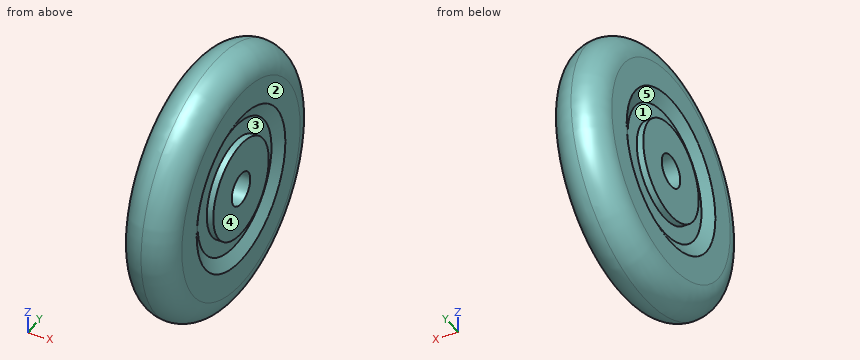
```python
from build123d import *


with BuildPart() as f1:
    # F0 (on Front) → F1 (revolve)
    with BuildSketch(Plane.XZ):
        with BuildLine():
            Line((-12.7, 7.9375), (0, 7.9375))
            Line((0, 7.9375), (12.7, 7.9375))
            Line((12.7, 7.9375), (12.7, 23.8125))
            Line((12.7, 23.8125), (9.525, 23.8125))
            Line((9.525, 23.8125), (9.525, 31.75))
            Line((9.525, 31.75), (12.7, 38.1))
            Line((12.7, 38.1), (12.7, 50.8))
            ThreePointArc((12.7, 50.8), (8.980256, 59.780256), (0, 63.5))
            ThreePointArc((0, 63.5), (-8.980256, 59.780256), (-12.7, 50.8))
            Line((-12.7, 50.8), (-12.7, 38.1))
            Line((-12.7, 38.1), (-9.525, 31.75))
            Line((-9.525, 31.75), (-9.525, 23.8125))
            Line((-9.525, 23.8125), (-12.7, 23.8125))
            Line((-12.7, 23.8125), (-12.7, 7.9375))
        make_face()
    revolve(axis=Axis((-3.268924, 0, 0), (1, 0, 0)))


solid = f1.part
```
Geometry check sheet. Reference: the model listing, model coordinates, mm. Face numbers are marked on the shaded views. A direction names the side the tool comes from. Give positions to 0.01 mm unless a question says otherwise; leave off trailing zeros. Loops run counter-clockwise (first coordinate to the right, second up) from the corner with the lowest first, then second, coordinate; pieces in that order, holes last. Notation, with made-up numbers: M 42.5,43.5 L 54.5,43.5 A17 cw 54.5,69.5 Z; hole C -15,16.5 d11. An arc over 180 degrees is marked long. Write item = value, one per line. Start each with the question number.
1. Draft check along Z on the marked faces 4 and 5. Enter one of: +Z half, -Z half, draft (parallel to the pull), parting line (faces both ways), or undercut.
2. Tool access check on the marked faces 1, 2 and 3. Record the directions out of +Z, -Z, +X, -X, +Y, -Y that give a thin tool (end or side, any length) a straight path to the whole face; none if there is none.
3. Section check A-A, the plane x = 6.25. Enter the section's corners in (y, z) (1 decimal).
4. Go/stop test with flat-tipped pins: P1, Ø8, axis at x = -9.5, y = 21, coming from the +Z side; P2, Ø6, axis at x = 1, y = -20.5, coming from the -Z side; P3, Ø12, axis at x = -4, y = 36, coming from the +Z side; P4, Ø20.5, axis at y = 0, z = 0, coming from the -X side. Record where each tip stops, or that it passes through.
5. Thickness scan on probe 1 along Z at (x, y) = (-0.25, 0); probe 2 along Z at (x, y) = (-10.25, 2); probe 3 along X at (y, z) = (20, -15) (3 decimals). Record the ranges inside material, lowest first.
Values follow:
q1.face_4 = draft
q1.face_5 = undercut
q2.face_1 = -X
q2.face_2 = +Z, -Z, +X, +Y, -Y
q2.face_3 = +X
q3.outline = C 0,0 d123.7; hole C 0,0 d15.9
q4.P1 = 58.99
q4.P2 = -61.02
q4.P3 = 55.6
q4.P4 = -12.7
q5.probe_1 = -63.5 to -7.94, 7.94 to 63.5
q5.probe_2 = -58.26 to -33.14, -23.73 to -7.68, 7.68 to 23.73, 33.14 to 58.26
q5.probe_3 = -9.525 to 9.525
